Check sheet for the drawn part. Datum: minimum x, y, z corner. Units: mm. A direction names the side the tool comes from. Give positions to 0.01 mm unless a question says otherwise; leave off trailing zeros. Order: outer loops, then holes, each group sorted by start corner. A loop starts at its lowest first (then second) coordinate and runs counter-clockwise, first axis right, second up. Notation, with made-up numbers: (75.25, 29) -> (126.25, 29) arc R26 cw to (126.25, 50) -> close; hole circle Ø1 at (-7.75, 32.5). An arc over 180 degrees is marked (long way). One line per question, with ' | ' between items. Start each with the question number.
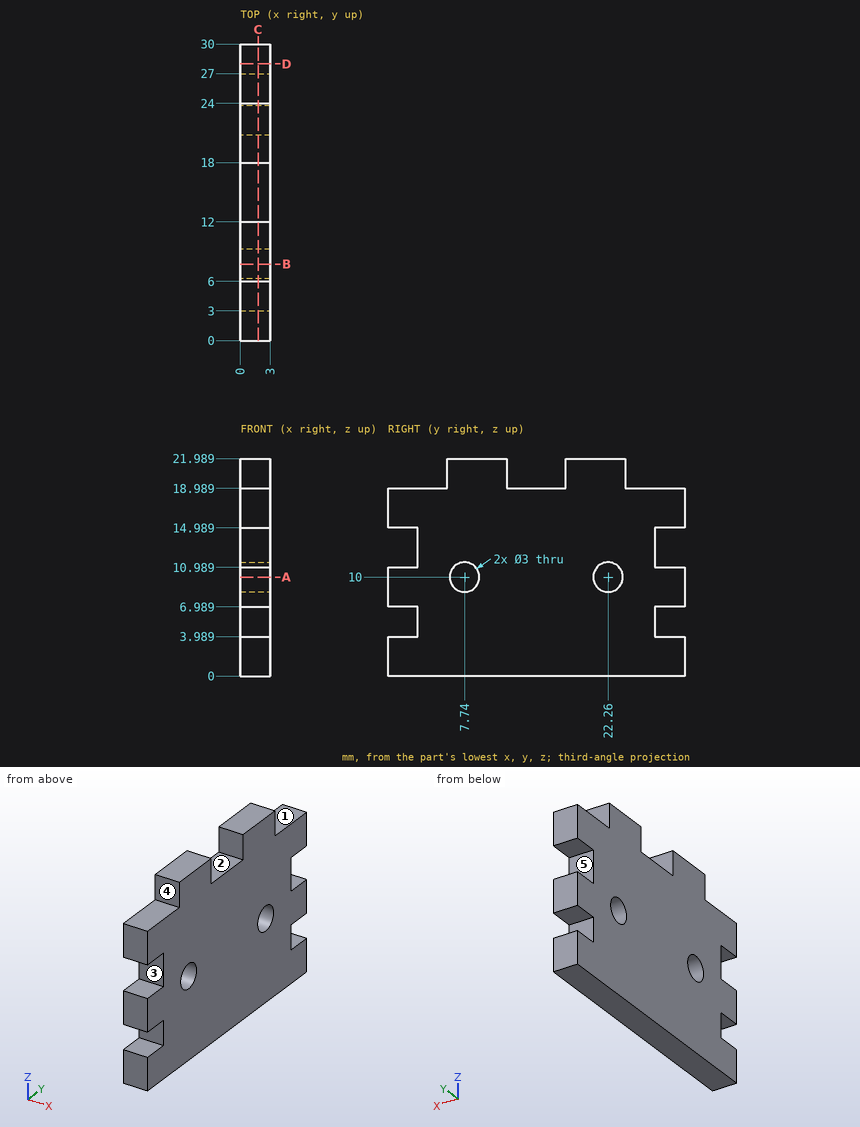
1. Cross-section at D-D on y = 28. Record the boundary of the cut face in (x, z).
2. Cross-section at B-B on y = 7.74. Record the boundary of the cut face in (x, z).
3. Go/stop test with flat-tipped pins: pin 1 (0.9 mm diameter, centred on x = 1.5, y = 14.5, fed in from +Z); pin 2 (1.5 mm diameter, centred on x = 1.5, z = 14, fed in from -Y); pin 3 (1.5 mm diameter, centred on x = 2, z = 20.5, fed in from +Y). Record where each tip stops, or that it passes through.
4. Scan lines: probe 1 along Y at (x, z) = (1.6, 10); probe 2 along Z at (x, y) = (0.8, 27.5); probe 3 along Y at (x, z) = (1.5, 8.75). Record each from-to range of solid material in increasing order.
5. Tool access check on the marked faces 1, 2, 3, 4 and 5. Record the directions out of +Z, -Z, +X, -X, +Y, -Y that give a thin tool (end or side, any length) a straight path to the whole face; none if there is none.
6. Cross-section at C-C on x = 1.8. Give the number of separate pieces and of enclosed holes in the cut face.
7. Cross-section at A-A on z = 10. Record the boundary of the cut face in (x, y).
Response values:
1) outline: (0, 0) -> (3, 0) -> (3, 3.99) -> (0, 3.99) -> close; (0, 6.99) -> (3, 6.99) -> (3, 10.99) -> (0, 10.99) -> close; (0, 14.99) -> (3, 14.99) -> (3, 18.99) -> (0, 18.99) -> close
2) outline: (0, 0) -> (3, 0) -> (3, 8.5) -> (0, 8.5) -> close; (0, 11.5) -> (3, 11.5) -> (3, 21.99) -> (0, 21.99) -> close
3) pin 1: stops at z = 18.99 | pin 2: stops at y = 3 | pin 3: stops at y = 24
4) probe 1: y = 0 to 6.24, 9.24 to 20.76, 23.76 to 30 | probe 2: z = 0 to 3.99, 6.99 to 10.99, 14.99 to 18.99 | probe 3: y = 0 to 6.91, 8.57 to 21.43, 23.09 to 30
5) face 1: +Z, +X, -X, +Y | face 2: +Z, +X, -X | face 3: +X, -X, -Y | face 4: +Z, +X, -X, -Y | face 5: +X, -X, +Y
6) separate pieces: 1 | enclosed holes: 2
7) outline: (0, 0) -> (3, 0) -> (3, 6.24) -> (0, 6.24) -> close; (0, 9.24) -> (3, 9.24) -> (3, 20.76) -> (0, 20.76) -> close; (0, 23.76) -> (3, 23.76) -> (3, 30) -> (0, 30) -> close
